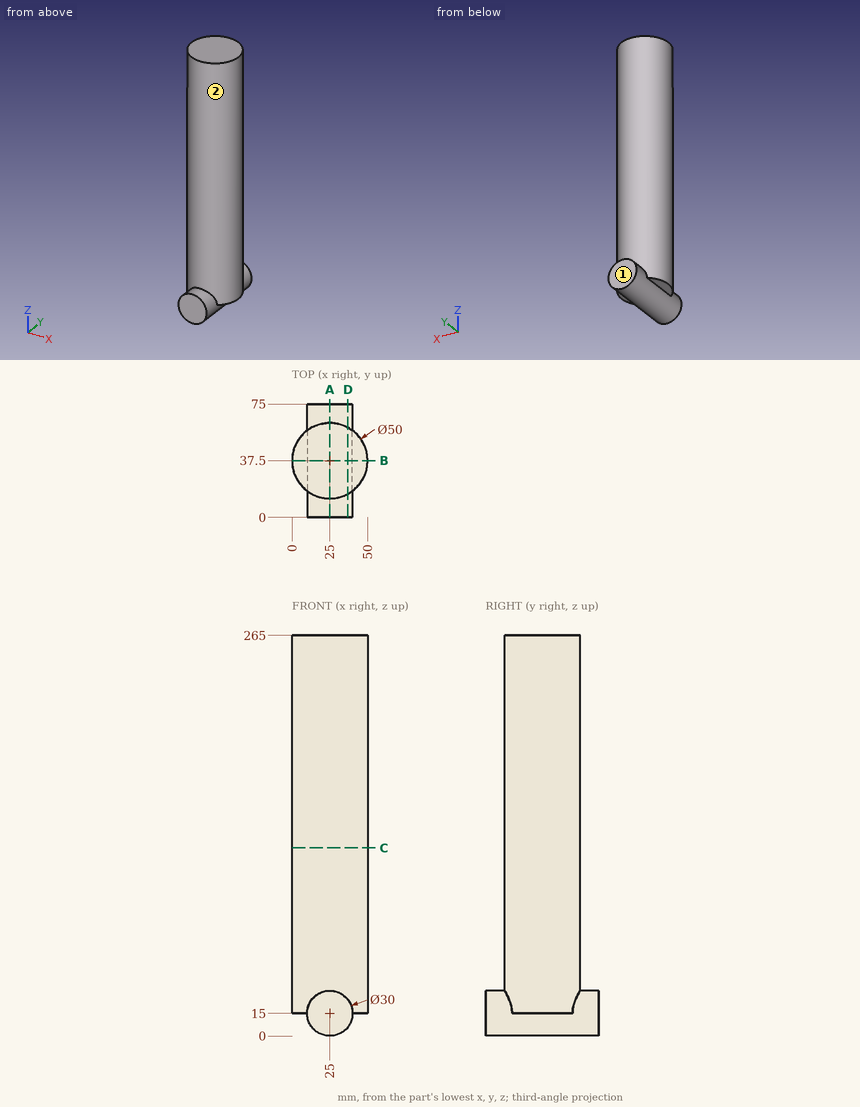
For this review, use the dimensioned drawing (mm, ordinates from the lowest corner) and the shaded views. A direction names the side the tool comes from. Coordinates: 2 decimals unless noted, no trailing zeros. Loops run counter-clockwise (first coordinate to the right, second up) from the corner with the lowest first, then second, coordinate; pieces in that order, holes last. Notation, with made-up numbers: (50, -39) -> (58, -39) arc R17 ccw to (58, -15) -> close; hole circle Ø4 at (53.25, 60). An arc over 180 degrees is marked (long way). Use a Markdown table: item, result. Add a question column.
1. Add section C-C on z = 124.5. Write out the cut boundary in (x, y).
2. Add section D-D on x = 37. Write out the cut boundary in (y, z).
3. Add section A-A on x = 25. Write out the cut boundary in (y, z), plus the area to 3 significant figures.
4. Add section B-B on y = 37.5. Write out the cut boundary in (x, z).
5. Clearance check with flat-ended pins moving along their axes: pin 1 Ø1 at (x, z) = (25, 208.5) entering from -Y; pin 2 Ø3 at (x, y) = (4.5, 30) entering from -Z; pin 3 Ø3 at (x, y) = (25.5, 15) entering from -Z; pin 4 Ø6 at (x, y) = (13.5, 64) entering from +Z. State where each tip first meets the part, or that it passes through.
6. Machinability: for the marked faces 1 and 2, which of the approach directions +Z, -Z, +X, -X, +Y, -Y give a long, thin tool a straight path to every point of the face, cutting with its end or side? Answer none if there is none.
7. To check wall thickness, follow line 1 (Z direction, x = 47.5, y = 41); line 2 (Z direction, x = 32, y = 35.5); line 3 (Y direction, x = 10.5, z = 87.5). State the ranges of each line that lie inside material, in increasing order.
Returned:
| question | item | result |
|---|---|---|
| 1 | outline | circle Ø50 at (25, 37.5) |
| 2 | outline | (0, 6) -> (75, 6) -> (75, 24) -> (59.43, 24) -> (59.43, 265) -> (15.57, 265) -> (15.57, 24) -> (0, 24) -> close |
| 3 | outline | (0, 0) -> (75, 0) -> (75, 30) -> (62.5, 30) -> (62.5, 265) -> (12.5, 265) -> (12.5, 30) -> (0, 30) -> close |
| 3 | area | 14,000 mm² |
| 4 | outline | (0, 15) -> (10, 15) arc R15 ccw to (40, 15) -> (50, 15) -> (50, 265) -> (0, 265) -> close |
| 5 | pin 1 | stops at y = 12.5 |
| 5 | pin 2 | stops at z = 15 |
| 5 | pin 3 | stops at z = 0 |
| 5 | pin 4 | stops at z = 27.36 |
| 6 | face 1 | +Z, -Z, +X, -X, +Y |
| 6 | face 2 | +Z |
| 7 | line 1 | z = 15 to 265 |
| 7 | line 2 | z = 1.73 to 265 |
| 7 | line 3 | y = 17.13 to 57.87 |
